Job drawing, mm, ordinate dimensions from the low corner. One solid piece. Round coordinates to 2 decimals unless told otherwise and drop trailing zeros. Order: outer loops, then holes, each group sorted by start corner. A loop starts at its lowest first (then second) coordinate and runs counter-clockwise, first axis right, second up. Notation, with made-up numbers: (50, 72) -> (61, 72) arc R32 ccw to (61, 101) -> close; hole circle Ø7 at (0, -20.75). An arc over 180 degrees is marked (long way). Return JSON: item names as keys, results as strings. Group by question number.
Q1. Cut at A-A (y = 1.25). Write the cut outline in (x, z).
Q2. Cut at B-B (y = 7.5). Write the cut outline in (x, z) (1 decimal).
Q3. Probe line 1 along X through (y, z) = (5, 1.9); line 2 along X through (y, z) = (4.75, 1.2); line 3 along Z through (x, y) = (3.35, 7.75) (1 decimal). List the from-to ranges inside material, lowest first.
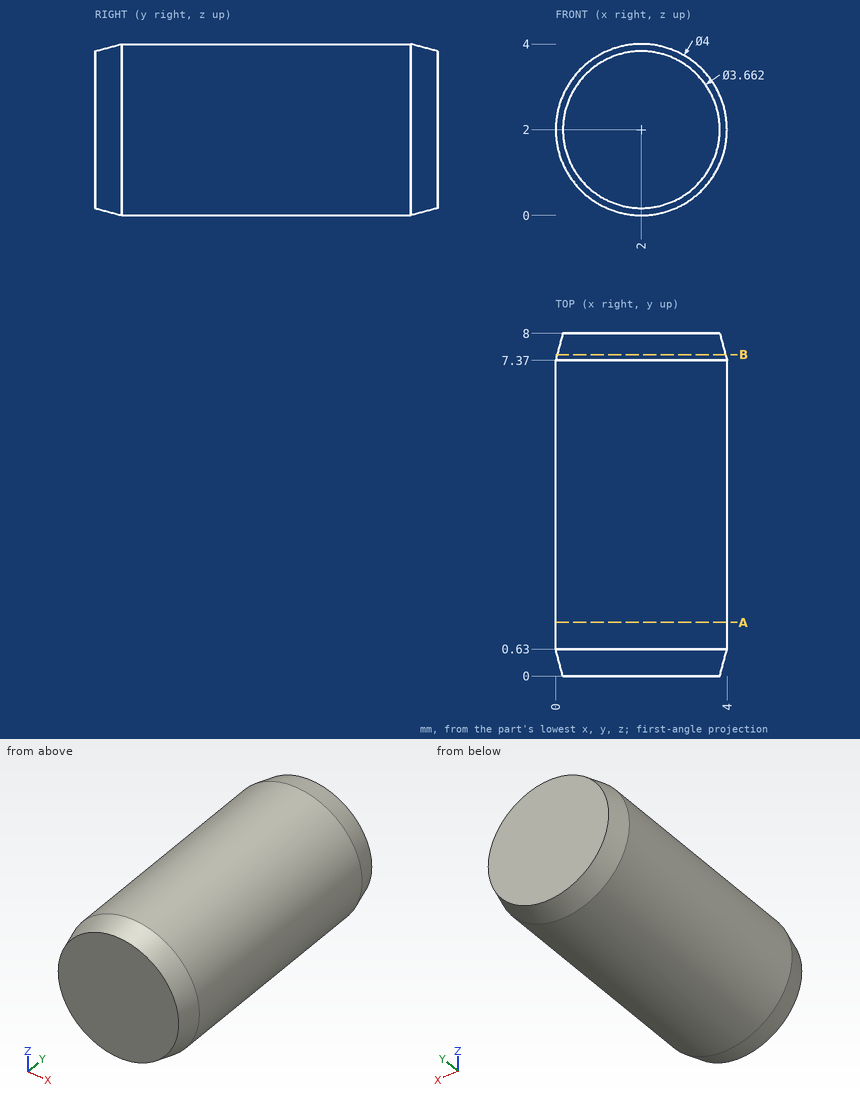
Solution:
{
 "1": {"outline": "circle Ø4 at (2, 2)"},
 "2": {"outline": "circle Ø3.9 at (2, 2)"},
 "3": {"line 1": "x = 0 to 4", "line 2": "x = 0.17 to 3.83", "line 3": "z = 0.7 to 3.3"}
}
